Read the model definition and answer for the solid it produces. Units are mm, in the model's axes. Face numbers are marked on the shaded views. A direction names the side the tool comes from. Coordinates: 2 decimals unless noted, no trailing zeros. Order: outer loops, then holes, each group sorted by start corner. A loop starts at its lowest first (then second) coordinate and runs counter-clockwise, first axis right, second up.
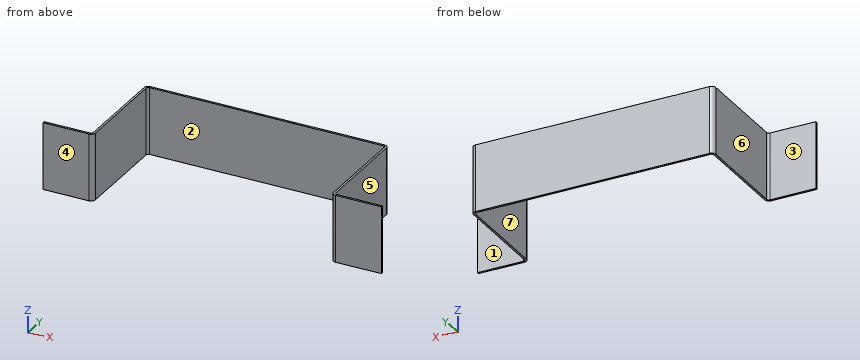
Autodesk Inventor part; units mm, degrees
ref_plane "YZ Plane" through (0, 0, 0) normal (1, 0, 0) x (0, 1, 0)
ref_plane "XZ Plane" through (0, 0, 0) normal (0, 1, 0) x (-1, 0, 0)
ref_plane "XY Plane" through (0, 0, 0) normal (0, 0, 1) x (1, 0, 0)
sketch "Sketch1" plane through (0, 0, 0) normal (0, 1, 0) x (-1, 0, 0)
  line L0 (0, 0) -> (180.975, 0)
  line L1 (180.975, 0) -> (180.975, -50.8)
  line L2 (180.975, -50.8) -> (0, -50.8)
  line L3 (0, -50.8) -> (0, 0)
  dimension "d0" = 180.975
  dimension "d1" = 50.8
extrude "Plate1" add sketch "Sketch1" along normal blind 1.5875
sketch "Sketch2" plane through (0, 0, 0) normal (1, 0, 0) x (0, 1, 0)
  line L0 (0, -50.8) -> (0, 0)
  line L1 (0, 0) -> (-76.0603, 0)
  line L2 (-76.0603, 0) -> (-76.0603, -50.8)
  line L3 (-76.0603, -50.8) -> (0, -50.8)
edge flange "Flange1" height 77.6478 angle 90 thickness 1.5875 bend radius 1.5875 thickness toward (1, 0, 0) relief straight relief width 1.5875 relief depth 0.7937 corner gap 1.5875 corner form 0 edges at (0, 0, -25.4) (-180.975, 0, -25.4) wall of the first edge with corners at (0, 0, -50.8) (0, 0, 0) (0, -76.0603, 0) (0, -76.0603, -50.8)
bend "Bend1"
corner "Corner1"
sketch "Sketch3" plane through (1.5875, -76.0603, -50.8) normal (0, -1, 0) x (1, 0, 0)
  line L0 (0, 50.8) -> (0, 0)
  line L1 (0, 0) -> (36.5125, 0)
  line L2 (36.5125, 0) -> (36.5125, 50.8)
  line L3 (36.5125, 50.8) -> (0, 50.8)
edge flange "Flange2" height 38.1 angle 90 thickness 1.5875 bend radius 1.5875 thickness toward (0, -1, 0) relief straight relief width 1.5875 relief depth 0.7937 corner gap 1.5875 corner form 0 edges at (1.5875, -76.0603, -25.4) (-182.5625, -76.0603, -25.4) wall of the first edge with corners at (1.5875, -76.0603, 0) (1.5875, -76.0603, -50.8) (38.1, -76.0603, -50.8) (38.1, -76.0603, 0)
bend "Bend2"
corner "Corner2"
equation "\"d3\" = BendReliefWidth"
equation "\"d4\" = BendReliefDepth"
equation "\"d5\" = MinimumRemnant"
equation "\"d6\" = BendRadius"
equation "\"d9\" = BendRadius"
equation "\"d10\" = CornerReliefSize"
equation "\"d11\" = GapSize"
equation "\"d12\" = JacobiRadiusSize"
equation "\"d13\" = BendReliefWidth"
equation "\"d14\" = BendReliefDepth"
equation "\"d15\" = MinimumRemnant"
equation "\"d16\" = BendRadius"
equation "\"d19\" = BendRadius"
equation "\"d20\" = CornerReliefSize"
equation "\"d21\" = GapSize"
equation "\"d22\" = JacobiRadiusSize"
equation "\"BendRadius\" = Thickness"
equation "\"BendReliefWidth\" = Thickness"
equation "\"BendReliefDepth\" = 0.5 * Thickness"
equation "\"CornerReliefSize\" = 4 * Thickness"
equation "\"MinimumRemnant\" = 2 * Thickness"
equation "\"TransitionRadius\" = BendRadius"
equation "\"JacobiRadiusSize\" = Thickness"
equation "\"GapSize\" = Thickness"
equation "\"d2\" = BendRadius"
properties part number "batteryHolder"
1) A cutting plane is placed at A-A, the plane y = -27.5. Determine the outline of the cut face in (x, z) (1 decimal), and give its area (3 significant figures).
A:
outline: (-182.6, -50.8) - (-181, -50.8) - (-181, 0) - (-182.6, 0) - close; (0, -50.8) - (1.6, -50.8) - (1.6, 0) - (0, 0) - close
area: 161 mm2
2) Straight lines are drawn through the part: line 1 (X direction, y = -12.5, z = -37) (1 decimal); line 2 (Y direction, x = -146.5, z = -11); line 3 (Y direction, x = -205.5, z = -45.5). For each, find the intervals that lie inside material, in ascending order.
A:
line 1: x = -182.6 to -181, 0 to 1.6
line 2: y = 0 to 1.59
line 3: y = -77.65 to -76.06
3) Determine the mould class of the marked faces 4, 5, 6 and 7 for opening direction X: pulls with the +X half, pulls with the -X half, needs draft (parallel to the pull), parting line crosses it, or undercut.
A:
face 4: needs draft
face 5: pulls with the +X half
face 6: pulls with the -X half
face 7: undercut
4) Flat-ended cylindrical pins translate along their axes: pin 1 Ø15 at (y, z) = (-36, -37.5) entering from -X; pin 2 Ø15 at (x, z) = (-51, -27.5) entering from -Y; pin 3 Ø6 at (x, y) = (-187, -20) entering from -Z; pin 4 Ø12 at (x, y) = (-1.5, -65) entering from +Z. Find the tip coordinate at first contact, or state that the pin passes through.
A:
pin 1: stops at x = -182.56
pin 2: stops at y = 0
pin 3: passes through
pin 4: stops at z = 0
5) Which of the six approach directions +Z, -Z, +X, -X, +Y, -Y give full straight-line access (tool end or side, diameter ignored) to the marked faces 1, 2 and 3?
A:
face 1: +Z, -Z, +X, +Y
face 2: +Z, -Z, -Y
face 3: +Z, -Z, -X, +Y
6) A cutting plane is placed at C-C, the plane x = -6. Determine the outline of the cut face in (y, z), and give its area (3 significant figures).
A:
outline: (0, -50.8) - (1.59, -50.8) - (1.59, 0) - (0, 0) - close
area: 80.6 mm2
